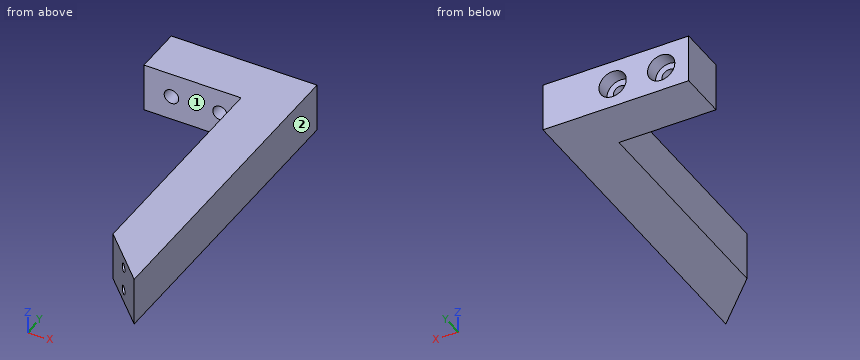
```python
from build123d import *

# Parameters (mm, degrees)
SKETCH1_W                                      = 38.1
SKETCH1_H                                      = 84.8
BOSS_EXTRUDE1_DEPTH                            = 6.35
SKETCH2_W                                      = 25.4
SKETCH2_H                                      = 72.1
CUT_EXTRUDE1_DEPTH                             = 13.7
CBORE_FOR_6_SOCKET_HEAD_CAP_SCREW1_D           = 3.7973
CBORE_FOR_6_SOCKET_HEAD_CAP_SCREW1_CBORE_D     = 7.14502
CBORE_FOR_6_SOCKET_HEAD_CAP_SCREW1_CBORE_DEPTH = 3.7051996
CUT_EXTRUDE2_DEPTH                             = 13.7
F_4_40_TAPPED_HOLE2_D                          = 2.2606
F_4_40_TAPPED_HOLE2_DEPTH                      = 7.59
F_4_40_TAPPED_HOLE2_TIP                        = 0.679152758


with BuildPart() as part:
    # Sketch1 → Boss-Extrude1 (new body, symmetric)
    with BuildSketch(Plane.XY):
        with Locations((19.05, -42.4)):
            Rectangle(SKETCH1_W, SKETCH1_H)
    extrude(amount=BOSS_EXTRUDE1_DEPTH, both=True)

    # Sketch2 → Cut-Extrude1 (cut, through all)
    with BuildSketch(Plane.XY.offset(6.35)):
        with Locations((12.7, -48.75)):
            Rectangle(SKETCH2_W, SKETCH2_H)
    extrude(amount=-CUT_EXTRUDE1_DEPTH, mode=Mode.SUBTRACT)

    # CBORE for #6 Socket Head Cap Screw1 (through all)
    with Locations(Plane(origin=(0, 0, 0), x_dir=(-1, 0, 0), z_dir=(0, 1, 0))):
        with Locations((-7.2, 0), (-19.9, 0)):
            CounterBoreHole(CBORE_FOR_6_SOCKET_HEAD_CAP_SCREW1_D / 2, CBORE_FOR_6_SOCKET_HEAD_CAP_SCREW1_CBORE_D / 2, CBORE_FOR_6_SOCKET_HEAD_CAP_SCREW1_CBORE_DEPTH)

    # Sketch9 → Cut-Extrude2 (cut, through all)
    with BuildSketch(Plane.XY.offset(6.35)):
        Polygon((38.1, -84.8), (24.4, -71.1), (24.4, -85.8), (38.1, -85.8), align=None)
    extrude(amount=-CUT_EXTRUDE2_DEPTH, mode=Mode.SUBTRACT)

    # #4-40 Tapped Hole2
    with Locations(Plane(origin=(-23.35, -23.35, 0), x_dir=(-0.707106781, 0.707106781, 0), z_dir=(-0.707106781, -0.707106781, 0))):
        with Locations((-77.923167287, 3.175), (-77.923167287, -3.175)):
            Hole(F_4_40_TAPPED_HOLE2_D / 2, depth=F_4_40_TAPPED_HOLE2_DEPTH)
            with Locations((0, 0, -(F_4_40_TAPPED_HOLE2_DEPTH + F_4_40_TAPPED_HOLE2_TIP / 2))):  # 118° drill point
                Cone(0, F_4_40_TAPPED_HOLE2_D / 2, F_4_40_TAPPED_HOLE2_TIP, mode=Mode.SUBTRACT)


solid = part.part
```
Source: CAD feature listing. Evaluate the final solid. Frame: model axes, mm. Face numbers are marked on the shaded views. A direction names the side the tool comes from. Give positions to 0.01 mm unless a question says otherwise; leave off trailing zeros. Order: outer loops, then holes, each group sorted by start corner. A loop starts at its lowest first (then second) coordinate and runs counter-clockwise, first axis right, second up.
(1) Access query for the marked faces 1 and 2. Directions: +Z, -Z, +X, -X, +Y, -Y. A direction counts if a zero-diameter tool reaches every point of the face in a straight line with its end or side. Return the directions, or none.
(2) Section query C-C (y = -9.5). Return the cut outline in (x, z).
(3) Section query A-A (z = 0). Return the cut outline in (x, y).
(4) Section query B-B (x = 19.9). Return the cut outline in (y, z), plus the area to 3 significant figures.
(5) Contact query for flat-ended pins moving along their axis: P1, Ø2, axis at y = -8.5, z = 4.5, coming from the -X side; P2, Ø2, axis at x = 8.5, z = -1.5, coming from the +Y side; P3, Ø1.5, axis at x = 6.5, z = -0.5, coming from the -Y side; P4, Ø1, axis at x = 24.5, z = 0.5, coming from the -Y side. Output: stop coordinate, or through.
(6) Material intervals for line 1 along Z through (x, y) = (7, -8); line 2 along Y through (x, z) = (14, 3); line 3 along Z through (x, y) = (7, -1), sorted ascending.
(7) Section query D-D (y = -51). Return the cut outline in (x, z).
Outcome:
1. face 1: +Z, -Z, -X, -Y
1. face 2: +Z, -Z, +X, +Y, -Y
2. outline: (0, -6.35) - (38.1, -6.35) - (38.1, 6.35) - (0, 6.35) - close; hole circle Ø3.8 at (7.2, 0); hole circle Ø3.8 at (19.9, 0)
3. outline: (0, -12.7) - (5.3, -12.7) - (5.3, -3.71) - (3.63, -3.71) - (3.63, 0) - (0, 0) - close; (9.1, -12.7) - (18, -12.7) - (18, -3.71) - (16.33, -3.71) - (16.33, 0) - (10.77, 0) - (10.77, -3.71) - (9.1, -3.71) - close; (21.8, -12.7) - (25.4, -12.7) - (25.4, -72.1) - (38.1, -84.8) - (38.1, 0) - (23.47, 0) - (23.47, -3.71) - (21.8, -3.71) - close
4. outline: (-12.7, -6.35) - (0, -6.35) - (0, -3.57) - (-3.71, -3.57) - (-3.71, -1.9) - (-12.7, -1.9) - close; (-12.7, 1.9) - (-3.71, 1.9) - (-3.71, 3.57) - (0, 3.57) - (0, 6.35) - (-12.7, 6.35) - close
4. area: 101 mm2
5. P1: stops at x = 0
5. P2: stops at y = -3.71
5. P3: passes through
5. P4: stops at y = -12.7
6. line 1: z = -6.35 to -1.89, 1.89 to 6.35
6. line 2: y = -12.7 to 0
6. line 3: z = -6.35 to -3.57, 3.57 to 6.35
7. outline: (25.4, -6.35) - (38.1, -6.35) - (38.1, 6.35) - (25.4, 6.35) - close
